Could you check a few things on this model? Use its own coordinates, in mm. Face numbers are marked on the shaded views. A direction names the side the tool comes from. Give positions to 0.01 mm unless a question says otherwise; leave off trailing zeros. Write each loop counter-clockwise with the first axis right and the second up, starting at its lowest first coordinate (ties: lowest second). Pieces come first, ordered by that corner, then holes. Notation, with made-up numbers: (65.25, -16) - (71.25, -16) arc R20 ccw to (71.25, 3) - close; hole circle Ø9 at (25.5, 51.25). An arc over 180 degrees is marked (long way). Answer as a JSON object with one key per item and string values. Group by question number.
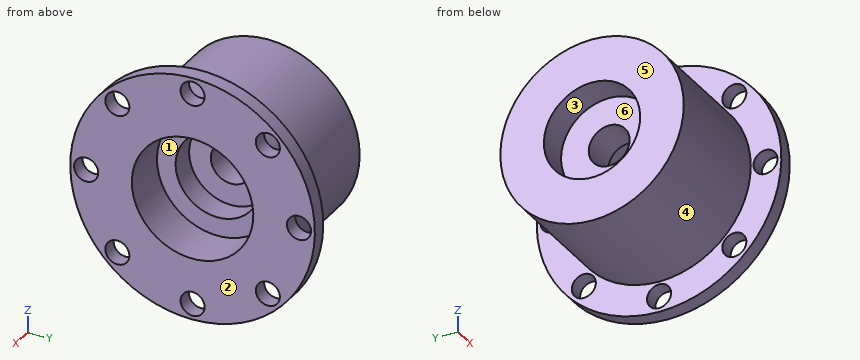
```python
from build123d import *

# Parameters (mm, degrees)
SKETCH1_R              = 38.1
BOSS_EXTRUDE1_DEPTH    = 38.1
SKETCH2_R              = 17.5
CUT_EXTRUDE1_DEPTH     = 10.25
F_25_0MM_DOWEL_HOLE1_D = 17
SKETCH14_R             = 38.1
SKETCH14_R_2           = 25.235346295
BOSS_EXTRUDE3_DEPTH    = 19.05
BOSS_EXTRUDE2_START    = -6.35
SKETCH7_R              = 50.8
SKETCH7_R_2            = 25.235346295
BOSS_EXTRUDE2_DEPTH    = 6.35
SKETCH8_R              = 20
CUT_EXTRUDE2_DEPTH     = 13
M8_CLEARANCE_HOLE1_D   = 10


with BuildPart() as part:
    # Sketch1 → Boss-Extrude1 (new body)
    with BuildSketch(Plane(origin=(0, 0, 0), x_dir=(0, 0, -1), z_dir=(1, 0, 0))):
        with Locations(Location((0, 0, 0), (0, 0, 180))):
            Circle(SKETCH1_R)
    extrude(amount=BOSS_EXTRUDE1_DEPTH)

    # Sketch2 → Cut-Extrude1 (cut)
    with BuildSketch(Plane(origin=(38.1, 0, 0), x_dir=(0, 0, -1), z_dir=(1, 0, 0))):
        Circle(SKETCH2_R)
    extrude(amount=-CUT_EXTRUDE1_DEPTH, mode=Mode.SUBTRACT)

    # Ø25.0mm Dowel Hole1 (through all)
    with Locations(Plane(origin=(27.85, 0, 0), x_dir=(0, 0, -1), z_dir=(1, 0, 0))):
        with Locations((0, 0)):
            Hole(F_25_0MM_DOWEL_HOLE1_D / 2)

    # Sketch14 → Boss-Extrude3 (add)
    with BuildSketch(Plane(origin=(38.1, 0, 0), x_dir=(0, 0, -1), z_dir=(1, 0, 0))):
        with Locations(Location((0, 0, 0), (0, 0, 180))):
            Circle(SKETCH14_R)
        with Locations(Location((0, 0, 0), (0, 0, 180))):
            Circle(SKETCH14_R_2, mode=Mode.SUBTRACT)
    extrude(amount=BOSS_EXTRUDE3_DEPTH)

    # Sketch7 → Boss-Extrude2 (add)
    with BuildSketch(Plane(origin=(57.15, 0, 0), x_dir=(0, 0, -1), z_dir=(1, 0, 0)).offset(BOSS_EXTRUDE2_START)):
        Circle(SKETCH7_R)
        with Locations(Location((0, 0, 0), (0, 0, 180))):
            Circle(SKETCH7_R_2, mode=Mode.SUBTRACT)
    extrude(amount=BOSS_EXTRUDE2_DEPTH)

    # Sketch8 → Cut-Extrude2 (cut)
    with BuildSketch(Plane.ZY):
        Circle(SKETCH8_R)
    extrude(amount=-CUT_EXTRUDE2_DEPTH, mode=Mode.SUBTRACT)

    # M8 Clearance Hole1 (through all)
    with Locations(Plane.ZY.offset(-50.8)):
        with Locations((-44.206688043, 0), (-31.258848889, 31.258848889), (0, 44.206688043), (31.258848889, 31.258848889), (44.206688043, 0), (31.258848889, -31.258848889), (0, -44.206688043), (-31.258848889, -31.258848889), (0, 0)):
            Hole(M8_CLEARANCE_HOLE1_D / 2)


solid = part.part
```
(1) If we mould it in two halves opening along Y, with no side actions, what happens to the marked faces 4, 5 and 6? For each: +Y half, -Y half, draft (parallel to the pull), parting line (faces both ways), or undercut.
(2) I want a section at D-D, the plane x = 18.5. Please give me the cut outline in (y, z).
(3) For the marked faces 1, 2 and 3, which set-ups out of +Z, -Z, +X, -X, +Y, -Y let a thin tool reach every point of the face, with its end or its side?
(4) I want a section at A-A, the plane y = 0. State how many separate pieces and enclosed holes the cut face has, and give its area (3 significant figures).
(5) I want a section at B-B, the plane z = 33. Please give me the cut outline in (x, y), and give its area (3 significant figures).
(6) Will these pins go through, and if not, where does the flat tip stop? P1, Ø6, axis at y = -44.21, z = 0, coming from the -X side; P2, Ø8, axis at x = 22, z = 8.5, coming from the -Y side; P3, Ø15, axis at y = 1, z = -5.5, coming from the +X side; P4, Ø6, axis at x = 10, y = -4, coming from the +Z side.
(7) I need wall thicknesses on L1, parallel to Y at x = 9.5, z = 0; L2, parallel to Y at x = 52.5, z = -28.5; L3, parallel to Y at x = 24, z = 0. Which ranges of each line are inside material? Lowest first, please.
Entries:
{
 "1": {"face 4": "parting line", "face 5": "draft", "face 6": "undercut"},
 "2": {"outline": "circle Ø76.2 at (0, 0); hole circle Ø17 at (0, 0)"},
 "3": {"face 1": "+X", "face 2": "+Z, -Z, +X, +Y, -Y", "face 3": "-X"},
 "4": {"separate pieces": "4", "enclosed holes": "0", "area": "2,300 mm^2"},
 "5": {"outline": "(0, -19.04) - (50.8, -19.04) - (50.8, -26.57) - (57.15, -26.57) - (57.15, 26.57) - (50.8, 26.57) - (50.8, 19.04) - (0, 19.04) - close; (50.8, -38.62) - (57.15, -38.62) - (57.15, -35.95) - (50.8, -35.95) - close; (50.8, 35.95) - (57.15, 35.95) - (57.15, 38.62) - (50.8, 38.62) - close", "area": "2,310 mm^2"},
 "6": {"P1": "through", "P2": "y = -37.83", "P3": "x = 27.85", "P4": "z = 38.09"},
 "7": {"L1": "-38.1 to -20, 20 to 38.1", "L2": "-42.05 to -35.43, -27.09 to 27.09, 35.43 to 42.05", "L3": "-38.1 to -8.5, 8.5 to 38.1"}
}
